The model under review builds one solid part; all positions refer to its coordinate system, in mm. Face numbers are marked on the shaded views. A direction names the side the tool comes from. Give positions to 0.01 mm unless a question says otherwise; leave off trailing zeros. Write each loop counter-clockwise with the first axis right and the second up, starting at its lowest first coordinate (ties: lowest second). Pieces come first, ordered by that corner, then holes. Notation, with made-up numbers: (66, 66.5) - (101, 66.5) arc R20 ccw to (101, 83.5) - close; hole circle Ø11 at (88.5, 69). An arc over 180 degrees is marked (long way). Write item = value, one per line.
```python
from build123d import *

# Parameters (mm, degrees)
F1_DEPTH = 14


with BuildPart() as f1:
    # F0 (on Front) → F1 (new body)
    with BuildSketch(Plane.XZ):
        with BuildLine():
            Line((-2.425778, 4.31487), (-5.591055, 9.240136))
            ThreePointArc((-5.591055, 9.240136), (-5.838921, 9.085538), (-6.082515, 8.924293))
            Line((-6.082515, 8.924293), (-2.917239, 3.999027))
            ThreePointArc((-2.917239, 3.999027), (-3.241561, 3.74096), (-3.543157, 3.456666))
            Line((-3.543157, 3.456666), (-7.967825, 7.290663))
            ThreePointArc((-7.967825, 7.290663), (-8.162095, 7.072496), (-8.350394, 6.849154))
            Line((-8.350394, 6.849154), (-3.925726, 3.015157))
            ThreePointArc((-3.925726, 3.015157), (-4.164205, 2.676172), (-4.373489, 2.318424))
            Line((-4.373489, 2.318424), (-9.699089, 4.750544))
            ThreePointArc((-9.699089, 4.750544), (-9.824026, 4.486482), (-9.941774, 4.219137))
            Line((-9.941774, 4.219137), (-4.616175, 1.787017))
            ThreePointArc((-4.616175, 1.787017), (-4.74949, 1.394576), (-4.849508, 0.992358))
            Line((-4.849508, 0.992358), (-10.644591, 1.825565))
            ThreePointArc((-10.644591, 1.825565), (-10.690072, 1.537), (-10.727731, 1.247311))
            Line((-10.727731, 1.247311), (-4.932648, 0.414104))
            ThreePointArc((-4.932648, 0.414104), (-4.95, 0), (-4.932648, -0.414104))
            Line((-4.932648, -0.414104), (-10.727731, -1.247311))
            ThreePointArc((-10.727731, -1.247311), (-10.690072, -1.537), (-10.644591, -1.825565))
            Line((-10.644591, -1.825565), (-4.849508, -0.992358))
            ThreePointArc((-4.849508, -0.992358), (-4.74949, -1.394576), (-4.616175, -1.787017))
            Line((-4.616175, -1.787017), (-9.941774, -4.219137))
            ThreePointArc((-9.941774, -4.219137), (-9.824026, -4.486482), (-9.699089, -4.750544))
            Line((-9.699089, -4.750544), (-4.373489, -2.318424))
            ThreePointArc((-4.373489, -2.318424), (-4.164205, -2.676172), (-3.925726, -3.015157))
            Line((-3.925726, -3.015157), (-8.350394, -6.849154))
            ThreePointArc((-8.350394, -6.849154), (-8.162095, -7.072496), (-7.967825, -7.290663))
            Line((-7.967825, -7.290663), (-3.543157, -3.456666))
            ThreePointArc((-3.543157, -3.456666), (-3.241561, -3.74096), (-2.917239, -3.999027))
            Line((-2.917239, -3.999027), (-6.082515, -8.924293))
            ThreePointArc((-6.082515, -8.924293), (-5.838921, -9.085538), (-5.591055, -9.240136))
            Line((-5.591055, -9.240136), (-2.425778, -4.31487))
            ThreePointArc((-2.425778, -4.31487), (-2.056304, -4.502678), (-1.672414, -4.65892))
            Line((-1.672414, -4.65892), (-3.321866, -10.276439))
            ThreePointArc((-3.321866, -10.276439), (-2.71605, -10.452898), (-2.100962, -10.593675))
            Line((-2.100962, -10.593675), (2.100962, -10.593675))
            ThreePointArc((2.100962, -10.593675), (2.71605, -10.452898), (3.321866, -10.276439))
            Line((3.321866, -10.276439), (1.672414, -4.65892))
            ThreePointArc((1.672414, -4.65892), (2.056304, -4.502678), (2.425778, -4.31487))
            Line((2.425778, -4.31487), (5.591055, -9.240136))
            ThreePointArc((5.591055, -9.240136), (5.838921, -9.085538), (6.082515, -8.924293))
            Line((6.082515, -8.924293), (2.917239, -3.999027))
            ThreePointArc((2.917239, -3.999027), (3.241561, -3.74096), (3.543157, -3.456666))
            Line((3.543157, -3.456666), (7.967825, -7.290663))
            ThreePointArc((7.967825, -7.290663), (8.162095, -7.072496), (8.350394, -6.849154))
            Line((8.350394, -6.849154), (3.925726, -3.015157))
            ThreePointArc((3.925726, -3.015157), (4.164205, -2.676172), (4.373489, -2.318424))
            Line((4.373489, -2.318424), (9.699089, -4.750544))
            ThreePointArc((9.699089, -4.750544), (9.824026, -4.486482), (9.941774, -4.219137))
            Line((9.941774, -4.219137), (4.616175, -1.787017))
            ThreePointArc((4.616175, -1.787017), (4.74949, -1.394576), (4.849508, -0.992358))
            Line((4.849508, -0.992358), (10.644591, -1.825565))
            ThreePointArc((10.644591, -1.825565), (10.690072, -1.537), (10.727731, -1.247311))
            Line((10.727731, -1.247311), (4.932648, -0.414104))
            ThreePointArc((4.932648, -0.414104), (4.95, 0), (4.932648, 0.414104))
            Line((4.932648, 0.414104), (10.727731, 1.247311))
            ThreePointArc((10.727731, 1.247311), (10.690072, 1.537), (10.644591, 1.825565))
            Line((10.644591, 1.825565), (4.849508, 0.992358))
            ThreePointArc((4.849508, 0.992358), (4.74949, 1.394576), (4.616175, 1.787017))
            Line((4.616175, 1.787017), (9.941774, 4.219137))
            ThreePointArc((9.941774, 4.219137), (9.824026, 4.486482), (9.699089, 4.750544))
            Line((9.699089, 4.750544), (4.373489, 2.318424))
            ThreePointArc((4.373489, 2.318424), (4.164205, 2.676172), (3.925726, 3.015157))
            Line((3.925726, 3.015157), (8.350394, 6.849154))
            ThreePointArc((8.350394, 6.849154), (8.162095, 7.072496), (7.967825, 7.290663))
            Line((7.967825, 7.290663), (3.543157, 3.456666))
            ThreePointArc((3.543157, 3.456666), (3.241561, 3.74096), (2.917239, 3.999027))
            Line((2.917239, 3.999027), (6.082515, 8.924293))
            ThreePointArc((6.082515, 8.924293), (5.838921, 9.085538), (5.591055, 9.240136))
            Line((5.591055, 9.240136), (2.425778, 4.31487))
            ThreePointArc((2.425778, 4.31487), (2.056304, 4.502678), (1.672414, 4.65892))
            Line((1.672414, 4.65892), (3.321866, 10.276439))
            ThreePointArc((3.321866, 10.276439), (2.819405, 10.425496), (2.310303, 10.55))
            Line((2.310303, 10.55), (0, 10.55))
            Line((0, 10.55), (-2.310303, 10.55))
            ThreePointArc((-2.310303, 10.55), (-2.819405, 10.425496), (-3.321866, 10.276439))
            Line((-3.321866, 10.276439), (-1.672414, 4.65892))
            ThreePointArc((-1.672414, 4.65892), (-2.056304, 4.502678), (-2.425778, 4.31487))
        make_face()
    extrude(amount=F1_DEPTH)


solid = f1.part
```
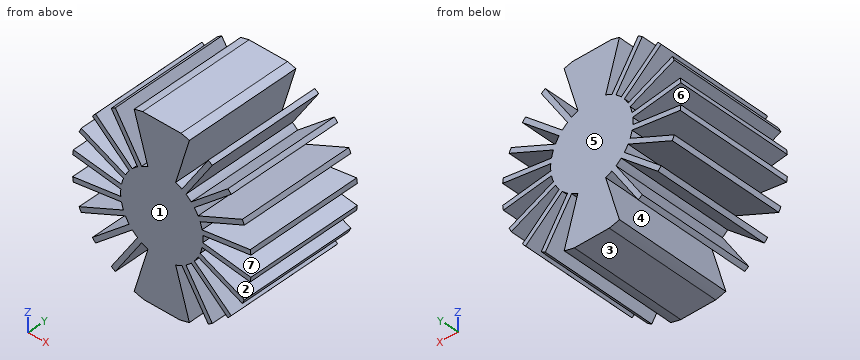
1. Machinability: for the marked faces 4, 5, 6 and 7, which of the approach directions +Z, -Z, +X, -X, +Y, -Y give a long, thin tool a straight path to every point of the face, cutting with its end or side? Answer none if there is none.
Findings below:
face_4 = +Y, -Y
face_5 = +Z, -Z, +X, -X, +Y
face_6 = -X, +Y, -Y
face_7 = +X, +Y, -Y
2. Take a section at C-C on z = 8.25. Give the boundary of the cut face in (x, y).
Findings below:
outline = (-5.65, -14) - (-4.95, -14) - (-4.95, 0) - (-5.65, 0) - close; (-2.73, -14) - (2.73, -14) - (2.73, 0) - (-2.73, 0) - close; (4.95, -14) - (5.65, -14) - (5.65, 0) - (4.95, 0) - close
3. For line 1 (X direction, y = -13.25, z = 5); line 2 (X direction, y = -7, z = 5.25); line 3 (Z direction, x = 7.75, y = -6.75), list the stretches that pass through material, from the lowest coordinate up. Write a range as from..to.
Findings below:
line_1 = -6.22..-5.32, -3.56..-2.87, -1.77..1.77, 2.87..3.56, 5.32..6.22
line_2 = -6.5..-5.61, -3.72..-3.03, -1.85..1.85, 3.03..3.72, 5.61..6.5
line_3 = -7.1..-6.33, -3.86..-3.22, -1.41..-0.82, 0.82..1.41, 3.22..3.86, 6.33..7.1
4. Take a section at B-B on x = 7.25. Give the boundary of the cut face in (y, z), and give its area (3 significant figures).
Findings below:
outline = (-14, -6.67) - (0, -6.67) - (0, -5.9) - (-14, -5.9) - close; (-14, -3.63) - (0, -3.63) - (0, -2.99) - (-14, -2.99) - close; (-14, -1.34) - (0, -1.34) - (0, -0.75) - (-14, -0.75) - close; (-14, 0.75) - (0, 0.75) - (0, 1.34) - (-14, 1.34) - close; (-14, 2.99) - (0, 2.99) - (0, 3.63) - (-14, 3.63) - close; (-14, 5.9) - (0, 5.9) - (0, 6.67) - (-14, 6.67) - close
area = 56.2 mm²
5. Take a section at A-A on z = -6.5. Give the boundary of the cut face in (x, y).
Findings below:
outline = (-7.95, -14) - (-7.06, -14) - (-7.06, 0) - (-7.95, 0) - close; (-4.52, -14) - (-3.83, -14) - (-3.83, 0) - (-4.52, 0) - close; (-2.21, -14) - (2.21, -14) - (2.21, 0) - (-2.21, 0) - close; (3.83, -14) - (4.52, -14) - (4.52, 0) - (3.83, 0) - close; (7.06, -14) - (7.95, -14) - (7.95, 0) - (7.06, 0) - close
6. Draft analysis for pull direction Z (two halves, no side actions). For the marked faces 1, 2 and 3, state which applies: +Z half, -Z half, draft (parallel to the pull), parting line (faces both ways), or undercut.
Findings below:
face_1 = draft
face_2 = undercut
face_3 = -Z half
